Work out the finished part from the listing and answer in its coordinate system (mm). A direction names the side the tool comes from. Coordinates: 2 decimals unless noted, no trailing zeros. Loops run counter-clockwise (first coordinate to the right, second up) from the corner with the lowest first, then second, coordinate; pieces in that order, holes last. Notation, with made-up numbers: (65, -37) -> (80, -37) arc R38 ccw to (80, 2) -> close; hole circle Ø11 at (-12.75, -20.5). An arc over 180 degrees is marked (long way). Use a Markdown table: item, result.
from build123d import *

# Parameters (mm, degrees)
EXTRUDE_1_DEPTH      = 23
SKETCH_2_W           = 5
SKETCH_2_H           = 20
CUT_EXTRUDE_1_DEPTH  = 5
SKETCH_3_R           = 1.5
CUT_EXTRUDE_2_DEPTH  = 106.470477522
SKETCH_5_W           = 70.883972197
SKETCH_5_H           = 5
CUT_EXTRUDE_3_DEPTH  = 5
SKETCH_6_W           = 26
SKETCH_6_H           = 5
EXTRUDE_2_DEPTH      = 23
CUT_EXTRUDE_4_REACH  = 112.223
SKETCH_7_W           = 21
SKETCH_7_H           = 14
SKETCH_9_W           = 42.093612699
SKETCH_9_H           = 5
CUT_EXTRUDE_6_DEPTH  = 5
CUT_EXTRUDE_7_REACH  = 103.079
SKETCH_10_W          = 7
SKETCH_10_H          = 13
SKETCH_12_W          = 12
SKETCH_12_H          = 5
EXTRUDE_4_DEPTH      = 14
EXTRUDE_5_DEPTH      = 5
CUT_EXTRUDE_8_REACH  = 107.632
SKETCH_14_R          = 1.45
SKETCH_15_W          = 5
SKETCH_15_H          = 5
CUT_EXTRUDE_9_DEPTH  = 6
CUT_EXTRUDE_5_REACH  = 112.223
SKETCH_8_R           = 1.5
SKETCH_16_W          = 9
SKETCH_16_H          = 10
EXTRUDE_6_DEPTH      = 5
SKETCH_17_W          = 9
SKETCH_17_H          = 10
CUT_EXTRUDE_10_DEPTH = 5


with BuildPart() as part:
    # 草圖1 → 填料-伸長1 (new body)
    with BuildSketch(Plane.XY):
        Polygon((-6.606934821, -8.392345722), (-6.606934821, -13.392345722), (-11.606934821, -13.392345722), (-11.606934821, 91.607654278), (-6.606934821, 91.607654278), (-6.606934821, 87.03530479), (-6.606934821, 81.216936273), (-6.606934821, -3.392345722), (24.393065179, -3.392345722), (24.393065179, -8.392345722), align=None)
    extrude(amount=EXTRUDE_1_DEPTH)

    # 草圖2 → 除料-伸長1 (cut)
    with BuildSketch(Plane(origin=(0, 0, 23), x_dir=(-1, 0, 0), z_dir=(0, 0, -1))):
        with Locations((9.106934821, 33.357654278)):
            Rectangle(SKETCH_2_W, SKETCH_2_H)
    extrude(amount=CUT_EXTRUDE_1_DEPTH, mode=Mode.SUBTRACT)

    # 草圖3 → 除料-伸長2 (cut, through all)
    with BuildSketch(Plane.XZ.offset(8.392345722)):
        with Locations((9.393065179, 11)):
            Circle(SKETCH_3_R)
    extrude(amount=-CUT_EXTRUDE_2_DEPTH, mode=Mode.SUBTRACT)

    # 草圖5 → 除料-伸長3 (cut)
    with BuildSketch(Plane.XY.offset(23)):
        with Locations((-11.04892092, -5.892345722)):
            Rectangle(SKETCH_5_W, SKETCH_5_H)
    extrude(amount=-CUT_EXTRUDE_3_DEPTH, mode=Mode.SUBTRACT)

    # 草圖6 → 填料-伸長2 (add)
    with BuildSketch(Plane(origin=(0, 0, 0), x_dir=(-1, 0, 0), z_dir=(0, 0, -1))):
        with Locations((-1.393065179, 89.107654278)):
            Rectangle(SKETCH_6_W, SKETCH_6_H)
    extrude(amount=-EXTRUDE_2_DEPTH)

    # 草圖7 → 除料-伸長4 (cut, up to next)
    with BuildSketch(Plane(origin=(0, 91.607654278, 0), x_dir=(1, 0, 0), z_dir=(0, 1, 0)), mode=Mode.PRIVATE) as cut_extrude_4_sk1:
        with Locations((3.893065179, -7)):
            Rectangle(SKETCH_7_W, SKETCH_7_H)
    cut_extrude_4_tool1 = extrude(cut_extrude_4_sk1.sketch, amount=-CUT_EXTRUDE_4_REACH, mode=Mode.PRIVATE) & part.part
    add(cut_extrude_4_tool1.solids().sort_by_distance((3.893065, 91.607654, 7))[0], mode=Mode.SUBTRACT)

    # 草圖9 → 除料-伸長6 (cut)
    with BuildSketch(Plane.XY.offset(23)):
        with Locations((-6.653741171, 89.107654278)):
            Rectangle(SKETCH_9_W, SKETCH_9_H)
    extrude(amount=-CUT_EXTRUDE_6_DEPTH, mode=Mode.SUBTRACT)

    # 草圖10 → 除料-伸長7 (cut, up to next)
    with BuildSketch(Plane.ZY.offset(11.606934821), mode=Mode.PRIVATE) as cut_extrude_7_sk1:
        with Locations((3.5, 72.107654278)):
            Rectangle(SKETCH_10_W, SKETCH_10_H)
    cut_extrude_7_tool1 = extrude(cut_extrude_7_sk1.sketch, amount=-CUT_EXTRUDE_7_REACH, mode=Mode.PRIVATE) & part.part
    add(cut_extrude_7_tool1.solids().sort_by_distance((-11.606935, 72.107654, 3.5))[0], mode=Mode.SUBTRACT)

    # 草圖12 → 填料-伸長4 (add)
    with BuildSketch(Plane(origin=(0, 0, 14), x_dir=(-1, 0, 0), z_dir=(0, 0, -1))):
        with Locations((-8.393065179, 89.107654278)):
            Rectangle(SKETCH_12_W, SKETCH_12_H)
    extrude(amount=EXTRUDE_4_DEPTH)

    # 草圖13 → 填料-伸長5 (add)
    with BuildSketch(Plane(origin=(0, 91.607654278, 0), x_dir=(1, 0, 0), z_dir=(0, 1, 0))):
        Polygon((2.393065179, -14), (-6.606934821, -14), (-6.606934821, 0), (-11.606934821, 0), (-11.606934821, -5), (-11.606934821, -18), (2.393065179, -18), align=None)
    extrude(amount=EXTRUDE_5_DEPTH)

    # 草圖14 → 除料-伸長8 (cut, up to next)
    with BuildSketch(Plane.ZY.offset(11.606934821), mode=Mode.PRIVATE) as cut_extrude_8_sk1:
        with Locations(Location((13, 76.607654278, 0), (0, 0, 270))):
            Circle(SKETCH_14_R)
    cut_extrude_8_tool1 = extrude(cut_extrude_8_sk1.sketch, amount=-CUT_EXTRUDE_8_REACH, mode=Mode.PRIVATE) & part.part
    # 草圖14 → 除料-伸長8 (cut, up to next)
    with BuildSketch(Plane.ZY.offset(11.606934821), mode=Mode.PRIVATE) as cut_extrude_8_sk2:
        with Locations(Location((13, 6.607654278, 0), (0, 0, 270))):
            Circle(SKETCH_14_R)
    cut_extrude_8_tool2 = extrude(cut_extrude_8_sk2.sketch, amount=-CUT_EXTRUDE_8_REACH, mode=Mode.PRIVATE) & part.part
    # 草圖14 → 除料-伸長8 (cut, up to next)
    with BuildSketch(Plane.ZY.offset(11.606934821), mode=Mode.PRIVATE) as cut_extrude_8_sk3:
        with Locations(Location((13, 61.607654278, 0), (0, 0, 270))):
            Circle(SKETCH_14_R)
    cut_extrude_8_tool3 = extrude(cut_extrude_8_sk3.sketch, amount=-CUT_EXTRUDE_8_REACH, mode=Mode.PRIVATE) & part.part
    # 草圖14 → 除料-伸長8 (cut, up to next)
    with BuildSketch(Plane.ZY.offset(11.606934821), mode=Mode.PRIVATE) as cut_extrude_8_sk4:
        with Locations(Location((13, 21.607654278, 0), (0, 0, 270))):
            Circle(SKETCH_14_R)
    cut_extrude_8_tool4 = extrude(cut_extrude_8_sk4.sketch, amount=-CUT_EXTRUDE_8_REACH, mode=Mode.PRIVATE) & part.part
    add(cut_extrude_8_tool1.solids().sort_by_distance((-11.606935, 76.607654, 13))[0], mode=Mode.SUBTRACT)
    add(cut_extrude_8_tool2.solids().sort_by_distance((-11.606935, 6.607654, 13))[0], mode=Mode.SUBTRACT)
    add(cut_extrude_8_tool3.solids().sort_by_distance((-11.606935, 61.607654, 13))[0], mode=Mode.SUBTRACT)
    add(cut_extrude_8_tool4.solids().sort_by_distance((-11.606935, 21.607654, 13))[0], mode=Mode.SUBTRACT)

    # 草圖15 → 除料-伸長9 (cut)
    with BuildSketch(Plane(origin=(0, 0, 0), x_dir=(-1, 0, 0), z_dir=(0, 0, -1))):
        with Locations((4.106934821, -5.892345722)):
            Rectangle(SKETCH_15_W, SKETCH_15_H)
    extrude(amount=-CUT_EXTRUDE_9_DEPTH, mode=Mode.SUBTRACT)

    # 草圖8 → 除料-伸長5 (cut, up to next)
    with BuildSketch(Plane(origin=(0, 91.607654278, 0), x_dir=(1, 0, 0), z_dir=(0, 1, 0)), mode=Mode.PRIVATE) as cut_extrude_5_sk1:
        with Locations(Location((8.393065179, -11, 0), (0, 0, 270))):
            Circle(SKETCH_8_R)
    cut_extrude_5_tool1 = extrude(cut_extrude_5_sk1.sketch, amount=-CUT_EXTRUDE_5_REACH, mode=Mode.PRIVATE) & part.part
    add(cut_extrude_5_tool1.solids().sort_by_distance((8.393065, 91.607654, 11))[0], mode=Mode.SUBTRACT)

    # 草圖16 → 填料-伸長6 (add)
    with BuildSketch(Plane(origin=(0, 0, 0), x_dir=(-1, 0, 0), z_dir=(0, 0, -1))):
        with Locations((2.106934821, 91.607654278)):
            Rectangle(SKETCH_16_W, SKETCH_16_H)
    extrude(amount=-EXTRUDE_6_DEPTH)

    # 草圖17 → 除料-伸長10 (cut)
    with BuildSketch(Plane.XY.offset(18)):
        with Locations((-2.106934821, 91.607654278)):
            Rectangle(SKETCH_17_W, SKETCH_17_H)
    extrude(amount=-CUT_EXTRUDE_10_DEPTH, mode=Mode.SUBTRACT)


solid = part.part
Q1. Consider line 1 (X direction, y = 87.8, z = 11); line 2 (Y direction, x = 2.5, z = 10); line 3 (Y direction, x = -8.5, z = 5.75). Determine where each line is inside the solid, lowest interval first. Write a range as [from, to].
Solved:
| item | result |
|---|---|
| line 1 | [-11.61, -6.61], [2.39, 6.89], [9.89, 14.39] |
| line 2 | [-8.39, -3.39], [86.61, 91.61] |
| line 3 | [-13.39, 65.61], [78.61, 96.61] |
Q2. Section D-D on x = -5 is taken. Determine the outline of the cut face in (y, z), and give its area (3 significant figures).
Solved:
| item | result |
|---|---|
| outline | (-8.39, 6) -> (-3.39, 6) -> (-3.39, 18) -> (-8.39, 18) -> close; (86.61, 0) -> (96.61, 0) -> (96.61, 5) -> (86.61, 5) -> close |
| area | 110 mm² |
Q3. For faces 4 (the flat face through (-1.607, -6, 3)), 5 (the cylindrical face through (10.78, -5.93, 10.43)), 6 (the flat face through (14.393, 89, 9)), determine the directions among +Z, -Z, +X, -X, +Y, -Y from which every point of the face is accessible in a straight line to the end or side of a thin tool.
Solved:
| item | result |
|---|---|
| face 4 | -Z, -Y |
| face 5 | -Y |
| face 6 | +Z, -Z, +X, +Y |
Q4. Determine the mould class of faces 1 (the flat face through (8, 89, 18)), 2 (the flat face through (-9, -13.392, 11)), 3 (the flat face through (-9, -3.392, 21)) for opening direction Y: pulls with the +Y half, pulls with the -Y half, needs draft (parallel to the pull), parting line crosses it, or undercut.
Solved:
| item | result |
|---|---|
| face 1 | needs draft |
| face 2 | pulls with the -Y half |
| face 3 | undercut |
Q5. Section B-B on x = 4 is taken. Determine the outline of the cut face in (y, z).
Solved:
| item | result |
|---|---|
| outline | (-8.39, 0) -> (-3.39, 0) -> (-3.39, 18) -> (-8.39, 18) -> close; (86.61, 0) -> (91.61, 0) -> (91.61, 18) -> (86.61, 18) -> close |
Q6. Section C-C on y = -6 is taken. Determine the outline of the cut face in (x, z), and give its area (3 significant figures).
Solved:
| item | result |
|---|---|
| outline | (-11.61, 0) -> (-6.61, 0) -> (-6.61, 6) -> (-1.61, 6) -> (-1.61, 0) -> (24.39, 0) -> (24.39, 18) -> (-11.61, 18) -> close; hole circle Ø3 at (9.39, 11) |
| area | 611 mm² |
Q7. Section A-A on z = 17 is taken. Determine the outline of the cut face in (x, y), and give its area (3 significant figures).
Solved:
| item | result |
|---|---|
| outline | (-11.61, -13.39) -> (-6.61, -13.39) -> (-6.61, -8.39) -> (24.39, -8.39) -> (24.39, -3.39) -> (-6.61, -3.39) -> (-6.61, 96.61) -> (-11.61, 96.61) -> close; (2.39, 86.61) -> (14.39, 86.61) -> (14.39, 91.61) -> (2.39, 91.61) -> close |
| area | 765 mm² |
Q8. Given pin 1 Ø12 at (y, z) = (79.5, 6) entering from +X; pin 2 Ø3.5 at (y, z) = (76.61, 13) entering from -X; pin 3 Ø9 at (x, z) = (5, 9) entering from -Y; pin 4 Ø2.5 at (x, y) = (-9, 90) entering from +Z, each flat-ended and moving along its own axis, determine where each tip first touches the part or whether it passes through.
Solved:
| item | result |
|---|---|
| pin 1 | x = -6.61 |
| pin 2 | x = -11.61 |
| pin 3 | y = -8.39 |
| pin 4 | z = 18 |
